Part model, mm, in its own coordinate system. Face numbers are marked on the shaded views. A direction names the side the tool comes from. Give positions to 0.01 mm unless a question says otherwise; leave off trailing zeros. Write each loop counter-clockwise with the first axis right and the second up, starting at its lowest first coordinate (ties: lowest second). Pieces come first, ordered by that corner, then holes. Notation, with made-up numbers: M 37.25,86 L 50.25,86 A12 ccw 50.25,98 Z; hole C 7,49.25 d8. An arc over 180 degrees is marked long. Use a Markdown table: item, result. Add a question column.
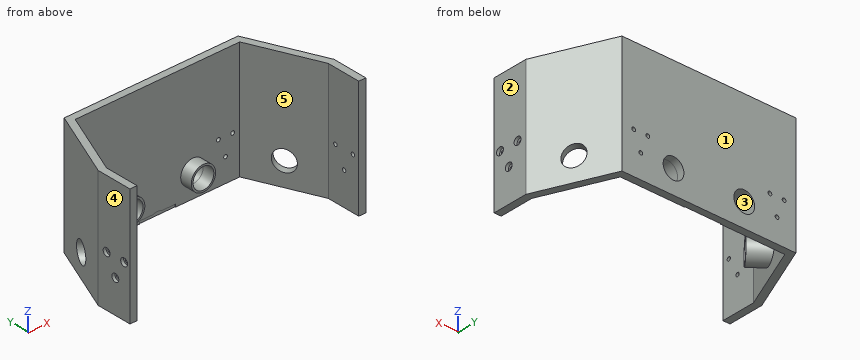
from build123d import *

# Parameters (mm, degrees)
SALIENTE_EXTRUIR1_DEPTH = 100
CORTAR_EXTRUIR1_REACH   = 170.346
CROQUIS3_R              = 8.8
CORTAR_EXTRUIR2_REACH   = 226.945
CROQUIS4_R              = 8.8
CORTAR_EXTRUIR3_DEPTH   = 0.5
CORTAR_EXTRUIR4_REACH   = 241.691
CROQUIS6_R              = 1.6
CROQUIS7_R              = 3.25
CORTAR_EXTRUIR5_DEPTH   = 2.5
CROQUIS11_R             = 10.3
CROQUIS11_R_2           = 8.8
SALIENTE_EXTRUIR2_DEPTH = 10
SALIENTE_EXTRUIR3_REACH = 201.802
CROQUIS12_R             = 10.3
CROQUIS12_R_2           = 8.8
CORTAR_EXTRUIR9_REACH   = 167.168
CROQUIS13_R             = 1.6


with BuildPart() as part:
    # Croquis1 → Saliente-Extruir1 (new body)
    with BuildSketch(Plane.XY):
        Polygon((-100, 25), (-100, -5), (-94, -5), (-94, 23.768453788), (-69.761533754, 80.324875029), (69.761533754, 80.324875029), (94, 23.768453788), (94, -5), (100, -5), (100, 25), (73.717910702, 86.324875029), (-73.717910702, 86.324875029), align=None)
    extrude(amount=SALIENTE_EXTRUIR1_DEPTH)

    # Croquis3 → Cortar-Extruir1 (cut, up to next)
    with BuildSketch(Plane(origin=(0, 86.324875029, 0), x_dir=(1, 0, 0), z_dir=(0, 1, 0)), mode=Mode.PRIVATE) as cortar_extruir1_sk1:
        with Locations(Location((-30, -20, 0), (0, 0, 270))):
            Circle(CROQUIS3_R)
    cortar_extruir1_tool1 = extrude(cortar_extruir1_sk1.sketch, amount=-CORTAR_EXTRUIR1_REACH, mode=Mode.PRIVATE) & part.part
    # Croquis3 → Cortar-Extruir1 (cut, up to next)
    with BuildSketch(Plane(origin=(0, 86.324875029, 0), x_dir=(1, 0, 0), z_dir=(0, 1, 0)), mode=Mode.PRIVATE) as cortar_extruir1_sk2:
        with Locations(Location((30, -20, 0), (0, 0, 270))):
            Circle(CROQUIS3_R)
    cortar_extruir1_tool2 = extrude(cortar_extruir1_sk2.sketch, amount=-CORTAR_EXTRUIR1_REACH, mode=Mode.PRIVATE) & part.part
    add(cortar_extruir1_tool1.solids().sort_by_distance((-30, 86.324875, 20))[0], mode=Mode.SUBTRACT)
    add(cortar_extruir1_tool2.solids().sort_by_distance((30, 86.324875, 20))[0], mode=Mode.SUBTRACT)

    # Cortar-Extruir2: up to this plane
    cortar_extruir2_end = Plane(origin=(-94, 23.768453788, 100), z_dir=(-0.9191450300180581, 0.3939192985791672, 0))
    # Croquis4 → Cortar-Extruir2 (cut, up to the surface)
    with BuildSketch(Plane(origin=(-87.479517168, 68.836107355, 0), x_dir=(0, 0, -1), z_dir=(-0.7858721058939679, 0.6183890629512945, 0)), mode=Mode.PRIVATE) as cortar_extruir2_sk1:
        with Locations(Location((-20, 9.96907102, 0), (0, 0, 270))):
            Circle(CROQUIS4_R)
    cortar_extruir2_tool1 = split(extrude(cortar_extruir2_sk1.sketch, amount=-CORTAR_EXTRUIR2_REACH, mode=Mode.PRIVATE), bisect_by=cortar_extruir2_end, keep=Keep.BOTH, mode=Mode.PRIVATE)
    cortar_extruir2 = cortar_extruir2_tool1.solids().sort_by_distance((-93.644282, 61.001693, 20))[0]
    add(cortar_extruir2, mode=Mode.SUBTRACT)

    # Simetría1: Cortar-Extruir2 across plane
    add(cortar_extruir2.mirror(Plane(origin=(0, 0, 0), x_dir=(0, 0, 1), z_dir=(1, 0, 0))), mode=Mode.SUBTRACT)

    # Croquis5 → Cortar-Extruir3 (cut)
    with BuildSketch(Plane.XZ.offset(-80.324875029)):
        with BuildLine():
            Line((14.875, 0), (15.175, 0))
            Line((15.175, 0), (15.175, 2.3))
            Line((15.175, 2.3), (3.784177586, 2.3))
            ThreePointArc((3.784177586, 2.3), (0, 3.1), (-3.784177586, 2.3))
            Line((-3.784177586, 2.3), (-15.175, 2.3))
            Line((-15.175, 2.3), (-15.175, 0))
            Line((-15.175, 0), (-14.875, 0))
            Line((-14.875, 0), (-14.875, 2))
            Line((-14.875, 2), (-3.720215048, 2))
            ThreePointArc((-3.720215048, 2), (0, 2.8), (3.720215048, 2))
            Line((3.720215048, 2), (14.875, 2))
            Line((14.875, 2), (14.875, 0))
        make_face()
        with BuildLine():
            Line((3.261901286, 0), (14.875, 0))
            Line((14.875, 0), (14.875, 2))
            Line((14.875, 2), (3.720215048, 2))
            ThreePointArc((3.720215048, 2), (0, 2.8), (-3.720215048, 2))
            Line((-3.720215048, 2), (-14.875, 2))
            Line((-14.875, 2), (-14.875, 0))
            Line((-14.875, 0), (-3.261901286, 0))
            ThreePointArc((-3.261901286, 0), (0, 0.8), (3.261901286, 0))
        make_face()
        with BuildLine():
            Line((-3.261901286, 0), (3.261901286, 0))
            ThreePointArc((3.261901286, 0), (0, 0.8), (-3.261901286, 0))
        make_face()
    extrude(amount=-CORTAR_EXTRUIR3_DEPTH, mode=Mode.SUBTRACT)

    # Croquis6 → Cortar-Extruir4 (cut, up to next)
    with BuildSketch(Plane.ZY.offset(100), mode=Mode.PRIVATE) as cortar_extruir4_sk1:
        with Locations(Location((43.227046774, 0.497681725, 0), (0, 0, 270))):
            Circle(CROQUIS6_R)
    cortar_extruir4_tool1 = extrude(cortar_extruir4_sk1.sketch, amount=-CORTAR_EXTRUIR4_REACH, mode=Mode.PRIVATE) & part.part
    # Croquis6 → Cortar-Extruir4 (cut, up to next)
    with BuildSketch(Plane.ZY.offset(100), mode=Mode.PRIVATE) as cortar_extruir4_sk2:
        with Locations(Location((27.863523387, 8.768453788, 0), (0, 0, 270))):
            Circle(CROQUIS6_R)
    cortar_extruir4_tool2 = extrude(cortar_extruir4_sk2.sketch, amount=-CORTAR_EXTRUIR4_REACH, mode=Mode.PRIVATE) & part.part
    # Croquis6 → Cortar-Extruir4 (cut, up to next)
    with BuildSketch(Plane.ZY.offset(100), mode=Mode.PRIVATE) as cortar_extruir4_sk3:
        with Locations(Location((43.227046774, 17.039225851, 0), (0, 0, 270))):
            Circle(CROQUIS6_R)
    cortar_extruir4_tool3 = extrude(cortar_extruir4_sk3.sketch, amount=-CORTAR_EXTRUIR4_REACH, mode=Mode.PRIVATE) & part.part
    cortar_extruir4_1 = cortar_extruir4_tool1.solids().sort_by_distance((-100, 0.497682, 43.227047))[0]
    add(cortar_extruir4_1, mode=Mode.SUBTRACT)
    cortar_extruir4_2 = cortar_extruir4_tool2.solids().sort_by_distance((-100, 8.768454, 27.863523))[0]
    add(cortar_extruir4_2, mode=Mode.SUBTRACT)
    cortar_extruir4_3 = cortar_extruir4_tool3.solids().sort_by_distance((-100, 17.039226, 43.227047))[0]
    add(cortar_extruir4_3, mode=Mode.SUBTRACT)
    cortar_extruir4 = cortar_extruir4_1 + cortar_extruir4_2 + cortar_extruir4_3  # Cortar-Extruir4 as one shape, for the pattern or mirror that repeats it

    # Croquis7 → Cortar-Extruir5 (cut)
    with BuildSketch(Plane.ZY.offset(100)):
        with Locations(Location((27.863523387, 8.768453788, 0), (0, 0, 270))):
            Circle(CROQUIS7_R)
        with Locations(Location((43.227046774, 0.497681725, 0), (0, 0, 270))):
            Circle(CROQUIS7_R)
        with Locations(Location((43.227046774, 17.039225851, 0), (0, 0, 270))):
            Circle(CROQUIS7_R)
    cortar_extruir5 = extrude(amount=-CORTAR_EXTRUIR5_DEPTH, mode=Mode.SUBTRACT)

    # Simetría2: Cortar-Extruir4, Cortar-Extruir5 across plane
    add(cortar_extruir4.mirror(Plane(origin=(0, 0, 0), x_dir=(0, 0, 1), z_dir=(1, 0, 0))), mode=Mode.SUBTRACT)
    add(cortar_extruir5.mirror(Plane(origin=(0, 0, 0), x_dir=(0, 0, 1), z_dir=(1, 0, 0))), mode=Mode.SUBTRACT)

    # Croquis11 → Saliente-Extruir2 (add)
    with BuildSketch(Plane.XZ.offset(-80.324875029)):
        with Locations(Location((-30, 20, 0), (0, 0, 90))):
            Circle(CROQUIS11_R)
        with Locations(Location((-30, 20, 0), (0, 0, 90))):
            Circle(CROQUIS11_R_2, mode=Mode.SUBTRACT)
        with Locations(Location((30, 20, 0), (0, 0, 90))):
            Circle(CROQUIS11_R)
        with Locations(Location((30, 20, 0), (0, 0, 90))):
            Circle(CROQUIS11_R_2, mode=Mode.SUBTRACT)
    extrude(amount=SALIENTE_EXTRUIR2_DEPTH)

    # Saliente-Extruir3: up to this plane
    saliente_extruir3_end = Plane(origin=(-94, 23.768453788, 100), z_dir=(-0.9191450300180581, 0.3939192985791672, 0))
    # Croquis12 → Saliente-Extruir3 (add, up to the surface)
    with BuildSketch(Plane(origin=(-63.903353991, 50.284435467, 0), x_dir=(0, 0, -1), z_dir=(-0.7858721058939679, 0.6183890629512945, 0)), mode=Mode.PRIVATE) as saliente_extruir3_sk1:
        with Locations(Location((-20, 9.96907102, 0), (0, 0, 90))):
            Circle(CROQUIS12_R)
        with Locations(Location((-20, 9.96907102, 0), (0, 0, 90))):
            Circle(CROQUIS12_R_2, mode=Mode.SUBTRACT)
    saliente_extruir3_tool1 = split(extrude(saliente_extruir3_sk1.sketch, amount=SALIENTE_EXTRUIR3_REACH, mode=Mode.PRIVATE), bisect_by=saliente_extruir3_end, keep=Keep.BOTH, mode=Mode.PRIVATE)
    add(saliente_extruir3_tool1.solids().sort_by_distance((-63.878865, 50.315557, 20))[0])

    # Croquis13 → Cortar-Extruir9 (cut, up to next)
    with BuildSketch(Plane.XZ.offset(-80.324875029), mode=Mode.PRIVATE) as cortar_extruir9_sk1:
        with Locations(Location((57.761533754, 20, 0), (0, 0, 270))):
            Circle(CROQUIS13_R)
    cortar_extruir9_tool1 = extrude(cortar_extruir9_sk1.sketch, amount=-CORTAR_EXTRUIR9_REACH, mode=Mode.PRIVATE) & part.part
    # Croquis13 → Cortar-Extruir9 (cut, up to next)
    with BuildSketch(Plane.XZ.offset(-80.324875029), mode=Mode.PRIVATE) as cortar_extruir9_sk2:
        with Locations(Location((51.761533754, 35, 0), (0, 0, 270))):
            Circle(CROQUIS13_R)
    cortar_extruir9_tool2 = extrude(cortar_extruir9_sk2.sketch, amount=-CORTAR_EXTRUIR9_REACH, mode=Mode.PRIVATE) & part.part
    # Croquis13 → Cortar-Extruir9 (cut, up to next)
    with BuildSketch(Plane.XZ.offset(-80.324875029), mode=Mode.PRIVATE) as cortar_extruir9_sk3:
        with Locations(Location((63.761533754, 35, 0), (0, 0, 270))):
            Circle(CROQUIS13_R)
    cortar_extruir9_tool3 = extrude(cortar_extruir9_sk3.sketch, amount=-CORTAR_EXTRUIR9_REACH, mode=Mode.PRIVATE) & part.part
    # Croquis13 → Cortar-Extruir9 (cut, up to next)
    with BuildSketch(Plane.XZ.offset(-80.324875029), mode=Mode.PRIVATE) as cortar_extruir9_sk4:
        with Locations(Location((-57.761533754, 20, 0), (0, 0, 270))):
            Circle(CROQUIS13_R)
    cortar_extruir9_tool4 = extrude(cortar_extruir9_sk4.sketch, amount=-CORTAR_EXTRUIR9_REACH, mode=Mode.PRIVATE) & part.part
    # Croquis13 → Cortar-Extruir9 (cut, up to next)
    with BuildSketch(Plane.XZ.offset(-80.324875029), mode=Mode.PRIVATE) as cortar_extruir9_sk5:
        with Locations(Location((-63.761533754, 35, 0), (0, 0, 270))):
            Circle(CROQUIS13_R)
    cortar_extruir9_tool5 = extrude(cortar_extruir9_sk5.sketch, amount=-CORTAR_EXTRUIR9_REACH, mode=Mode.PRIVATE) & part.part
    # Croquis13 → Cortar-Extruir9 (cut, up to next)
    with BuildSketch(Plane.XZ.offset(-80.324875029), mode=Mode.PRIVATE) as cortar_extruir9_sk6:
        with Locations(Location((-51.761533754, 35, 0), (0, 0, 270))):
            Circle(CROQUIS13_R)
    cortar_extruir9_tool6 = extrude(cortar_extruir9_sk6.sketch, amount=-CORTAR_EXTRUIR9_REACH, mode=Mode.PRIVATE) & part.part
    add(cortar_extruir9_tool1.solids().sort_by_distance((57.761534, 80.324875, 20))[0], mode=Mode.SUBTRACT)
    add(cortar_extruir9_tool2.solids().sort_by_distance((51.761534, 80.324875, 35))[0], mode=Mode.SUBTRACT)
    add(cortar_extruir9_tool3.solids().sort_by_distance((63.761534, 80.324875, 35))[0], mode=Mode.SUBTRACT)
    add(cortar_extruir9_tool4.solids().sort_by_distance((-57.761534, 80.324875, 20))[0], mode=Mode.SUBTRACT)
    add(cortar_extruir9_tool5.solids().sort_by_distance((-63.761534, 80.324875, 35))[0], mode=Mode.SUBTRACT)
    add(cortar_extruir9_tool6.solids().sort_by_distance((-51.761534, 80.324875, 35))[0], mode=Mode.SUBTRACT)


solid = part.part
1. Tool access for the marked faces 4 and 5: list every direction of +Z, -Z, +X, -X, +Y, -Y with a clear straight run to the whole face (end or side of a thin tool).
2. Flat gauge pins, fed straight in: pin 1 (23 mm diameter, centred on x = -30, z = 20, fed in from -Y); pin 2 (4 mm diameter, centred on y = 39, z = 10, fed in from +X); pin 3 (3 mm diameter, centred on y = 1, z = 42.5, fed in from +X). Where does each tip first touch, or does it go through?
3. Cut at C-C (z = 70.5). Write the cut outline in (x, y), then the cut area to 3 significant figures.
4. Cut at B-B (y = 73.5). Write the cut outline in (x, z), then the cut area to 3 significant figures.
5. Cut at A-A (x = 30). Write the cut outline in (y, z).
6. Cut at D-D (y = 32). Write the cut outline in (x, z), then the cut area to 3 significant figures.
7. Drill centre lines: probe 1 along X at (y, z) = (82.5, 35); probe 2 along X at (y, z) = (83.95, 35); probe 3 along X at (y, z) = (22, 58). Where is each one in solid material? Low to high. Write a range as [from, to].
8. Mould opens along X. For the marked faces 1, 2 and 3 say: released by +X, released by -X, zero draft, split by the parting line, or undercut.
A:
| question | item | result |
|---|---|---|
| 1 | face 4 | +Z, -Z, -X, +Y, -Y |
| 1 | face 5 | +Z, -Z, -Y |
| 2 | pin 1 | stops at y = 70.32 |
| 2 | pin 2 | stops at x = 94.86 |
| 2 | pin 3 | stops at x = 97.5 |
| 3 | outline | M -100,-5 L -94,-5 L -94,23.77 L -69.76,80.32 L 69.76,80.32 L 94,23.77 L 94,-5 L 100,-5 L 100,25 L 73.72,86.32 L -73.72,86.32 L -100,25 Z |
| 3 | area | 1,980 mm² |
| 4 | outline | M -79.21,0 L -72.69,0 L -72.69,100 L -79.21,100 Z; C -30,20 d20.6; C 30,20 d20.6; M 72.69,0 L 79.21,0 L 79.21,100 L 72.69,100 Z; hole C -30,20 d17.6; hole C 30,20 d17.6 |
| 4 | area | 1,490 mm² |
| 5 | outline | M 70.32,9.7 L 80.32,9.7 L 80.32,0 L 86.32,0 L 86.32,11.2 L 70.32,11.2 Z; M 70.32,28.8 L 86.32,28.8 L 86.32,100 L 80.32,100 L 80.32,30.3 L 70.32,30.3 Z |
| 6 | outline | M -97,0 L -90.47,0 L -90.47,100 L -97,100 Z; M 90.47,0 L 97,0 L 97,100 L 90.47,100 Z |
| 6 | area | 1,310 mm² |
| 7 | probe 1 | x = [-75.36, -65.36], [-62.16, -53.36], [-50.16, 50.16], [53.36, 62.16], [65.36, 75.36] |
| 7 | probe 2 | x = [-74.74, -65.36], [-62.16, -53.36], [-50.16, 50.16], [53.36, 62.16], [65.36, 74.74] |
| 7 | probe 3 | x = [-100, -94], [94, 100] |
| 8 | face 1 | zero draft |
| 8 | face 2 | released by +X |
| 8 | face 3 | undercut |
